Autodesk Inventor part; units mm, degrees
ref_plane "YZ Plane" through (0, 0, 0) normal (1, 0, 0) x (0, 1, 0)
ref_plane "XZ Plane" through (0, 0, 0) normal (0, 1, 0) x (-1, 0, 0)
ref_plane "XY Plane" through (0, 0, 0) normal (0, 0, 1) x (1, 0, 0)
sketch "Szkic1" plane through (0, 0, 0) normal (0, 0, 1) x (1, 0, 0)
  circle A0 centre (0.3365, 7.2308) radius 5
  circle A1 centre (-7.6635, 6.2308) radius 6
  circle A2 centre (5.3365, 0.2308) radius 6
  line L0 (-7.6635, 12.2308) -> (0.3365, 12.2308)
  line L1 (4.0398, 10.5902) -> (9.7804, 4.2621)
  line L2 (-10.1778, 0.783) -> (2.8222, -5.217)
  point P0 (0, 0)
  dimension "d0" = 13
  dimension "d1" = 6
  dimension "d2" = 7
  dimension "d3" = 5
  dimension "d4" = 10
  dimension "d5" = 12
  dimension "d6" = 12
extrude "Wyciągnięcie proste1" add sketch "Szkic1" along normal blind 3
hole "Otwór1" at (5.3365, 0.2308, 0) at (-7.6635, 6.2308, 0) direction (0, 0, 1) diameter 5 end through all
hole "Otwór2" at (0.3365, 7.2308, 0) direction (0, 0, 1) diameter 3 end through all
properties part number "mocowanie_sprezyny"
Geometry: final body of the model. Coordinates: model frame, mm. Coordinates: 2 decimals unless noted, no trailing zeros. Order: outer loops, then holes, each group sorted by start corner. A loop starts at its lowest first (then second) coordinate and runs counter-clockwise, first axis right, second up.
1) Section B-B (y = 6.5). Return loops of the section in (x, z), then the cut area to 3 significant figures.
Result sheet:
outline: (-13.66, 0) - (-10.15, 0) - (-10.15, 3) - (-13.66, 3) - close; (-5.18, 0) - (-0.97, 0) - (-0.97, 3) - (-5.18, 3) - close; (1.65, 0) - (7.75, 0) - (7.75, 3) - (1.65, 3) - close
area: 41.5 mm2
2) Section C-C (z = 2.55). Return loops of the section in (x, y), then the cut area to 3 significant figures.
Result sheet:
outline: (-10.18, 0.78) - (2.82, -5.22) arc R6 ccw to (9.78, 4.26) - (4.04, 10.59) arc R5 ccw to (0.34, 12.23) - (-7.66, 12.23) arc R6 ccw to start; hole circle Ø5 at (-7.66, 6.23); hole circle Ø3 at (0.34, 7.23); hole circle Ø5 at (5.34, 0.23)
area: 270 mm2
3) Section A-A (x = 3.5). Return loops of the section in (y, z).
Result sheet:
outline: (-5.48, 0) - (-1.47, 0) - (-1.47, 3) - (-5.48, 3) - close; (1.93, 0) - (11.1, 0) - (11.1, 3) - (1.93, 3) - close
4) Draft query along Y for faces 1 (the cylindrical face through (-5.223, 5.689, 1.521)), 2 (the flat face through (-1, 3, 0)), 3 (the cylindrical face through (-0.68, 6.13, 1.52)), 4 (the flat face through (6.87, 7.47, 1.48)). Return one class per face: released by +Y, released by -Y, zero draft, split by the parting line, or undercut.
Result sheet:
face 1: undercut
face 2: zero draft
face 3: undercut
face 4: released by +Y
5) Ray query, probe 1 along X at (y, z) = (6.75, 0.8); probe 2 along X at (y, z) = (6, 1.25); probe 3 along X at (y, z) = (-1.5, 2.65). Return the intervals inside material, ascending.
Result sheet:
probe 1: x = -13.64 to -10.11, -5.22 to -1.08, 1.76 to 7.52
probe 2: x = -13.66 to -10.15, -5.17 to -0.52, 1.19 to 8.2
probe 3: x = -5.23 to 3.53, 7.14 to 11.08
6) First-contact query: P1, Ø2.5, axis at x = 0.34, y = 7.23, coming from the +Z side. Flat tip, straight axial feed; report the tip coordinate or a pass-through.
Result sheet:
P1: passes through
7) Section D-D (y = 4). Return loops of the section in (x, z) (3 decimals), then the cut area to 3 significant figures.
Result sheet:
outline: (-13.233, 0) - (-8.792, 0) - (-8.792, 3) - (-13.233, 3) - close; (-6.535, 0) - (10.005, 0) - (10.005, 3) - (-6.535, 3) - close
area: 62.9 mm2
